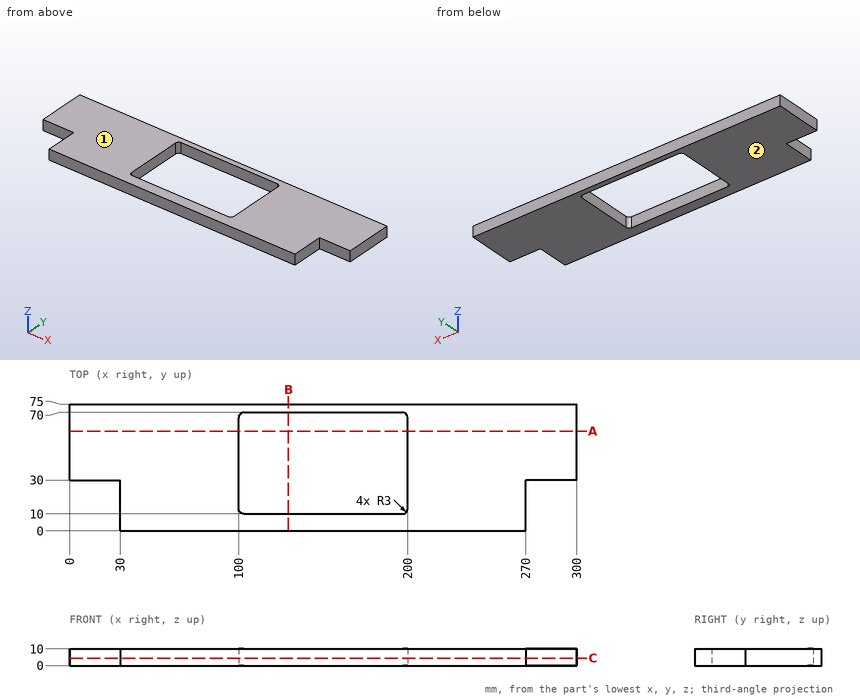
Can you work these out from the drawing? Everything is in mm from the part's minimum corner. Coordinates: 2 decimals unless noted, no trailing zeros. Loops run counter-clockwise (first coordinate to the right, second up) from the corner with the lowest first, then second, coordinate; pieces in that order, holes last. Notation, with made-up numbers: M 65,-17.5 L 94,-17.5 A23 ccw 94,10.5 Z; hole C 27,43.25 d8. An arc over 180 degrees is marked long. Put each result on its own line as item: value. Start each with the question number.
(1) I need wall thicknesses on line 1 (X direction, y = 41.5, z = 2); line 2 (X direction, y = 19.5, z = 1.75); line 3 (Y direction, x = 195.5, z = 5). Which ranges of each line are inside material? Lowest first, please. Write a range as from..to.
(2) Suppose I cut it at A-A on y = 59. Please give me the cut outline in (x, z).
(3) Will these pins go through, and if not, where does the flat tip stop? P1, Ø3, axis at y = 13, z = 5, coming from the +X side; P2, Ø3, axis at x = 279.5, z = 3, coming from the -Y side.
(4) Thinking about a two-plate mould opening in Z: for the marked faces 1 and 2, which applies, pulls with the +Z half, pulls with the -Z half, needs draft (parallel to the pull), parting line crosses it, or undercut?
(5) Suppose I cut it at B-B on x = 129.5. Please give me the cut outline in (y, z), then the cut area to 3 significant figures.
(6) Suppose I cut it at C-C on z = 4.5. Please give me the cut outline in (x, y).
Solutions:
1. line 1: x = 0..100, 200..300
1. line 2: x = 30..100, 200..270
1. line 3: y = 0..10, 70..75
2. outline: M 0,0 L 100,0 L 100,10 L 0,10 Z; M 200,0 L 300,0 L 300,10 L 200,10 Z
3. P1: stops at x = 270
3. P2: stops at y = 30
4. face 1: pulls with the +Z half
4. face 2: pulls with the -Z half
5. outline: M 0,0 L 10,0 L 10,10 L 0,10 Z; M 70,0 L 75,0 L 75,10 L 70,10 Z
5. area: 150 mm2
6. outline: M 0,30 L 30,30 L 30,0 L 270,0 L 270,30 L 300,30 L 300,75 L 0,75 Z; hole M 100,13 A3 ccw 103,10 L 197,10 A3 ccw 200,13 L 200,67 A3 ccw 197,70 L 103,70 A3 ccw 100,67 Z
